Could you check a few things on this model? Use its own coordinates, in mm. A direction names the side the tool comes from. Coordinates: 2 decimals unless noted, no trailing zeros. Order: outer loops, then holes, each group sorted by start corner. A loop starts at its lowest first (then second) coordinate and runs counter-clockwise, first axis right, second up. Notation, with made-up numbers: (72.25, 31) - (90.25, 31) arc R13 ccw to (90.25, 41) - close; hole circle Ø4 at (17.25, 10.5). An arc over 180 degrees is marked (long way). Answer as a JSON object with one key per item and string values. Group by question number.
(1) Will these pins go through, and if not, where does the flat tip stop? P1, Ø6.5, axis at x = 2, z = 2, coming from the +Y side (3 decimals); P2, Ø15, axis at x = 0, z = 0, coming from the -Y side; P3, Ø1, axis at y = 20, z = -20.5, coming from the -X side; P4, Ø11.5, axis at x = -218, z = -24, coming from the +Y side.
(2) Imagine slicing it at D-D, the plane x = -274.5. Write out the boundary of the cut face in (y, z).
(3) Imagine slicing it at B-B, the plane x = -215. Write out the boundary of the cut face in (y, z), and give its area (3 significant figures).
(4) Which directions (+Z, -Z, +X, -X, +Y, -Y) give clear straight access to the entire face, cutting with the end or side of a thin tool? Please do faces 1 (the flat face through (-152.4, 0, -19)), 2 (the flat face through (-255, 0, -50.8)), 3 (the flat face through (-355.6, 0, -19)).
(5) Imagine slicing it at C-C, the plane x = -107.5. Write out the boundary of the cut face in (y, z), and give its area (3 significant figures).
(6) Please list where these lines run through material, in increasing order: probe 1 along X at (y, z) = (-5.5, -23); probe 2 along X at (y, z) = (-14, -21); probe 3 along Z at (x, y) = (-151, 11.5).
from build123d import *

# Parameters (mm, degrees)
F1_DEPTH      = 31.75
F1_DEPTH_BACK = 31.75
F2_DEPTH      = 25.4
F2_DEPTH_BACK = 25.4
F3_R          = 6.35
F4_DEPTH      = 15.875
F5_R          = 6.35
F6_DEPTH      = 15.875


with BuildPart() as f1:
    # F0 (on Front) → F1 (new body, two sides)
    with BuildSketch(Plane.XZ) as f1_sk:
        with BuildLine():
            Line((0, -11.055585), (0, -6.35))
            ThreePointArc((0, -6.35), (4.490128, 4.490128), (-6.35, 0))
            Line((-6.35, 0), (-23.488146, 0))
            ThreePointArc((-23.488146, 0), (-25.145368, -0.220064), (-26.687727, -0.865004))
            Line((-26.687727, -0.865004), (-76.2, -29.747163))
            Line((-76.2, -29.747163), (-82.599162, -31.75))
            Line((-82.599162, -31.75), (-120.65, -31.75))
            ThreePointArc((-120.65, -31.75), (-123.825, -32.600739), (-126.149261, -34.925))
            ThreePointArc((-126.149261, -34.925), (-128.473523, -37.249261), (-131.648523, -38.1))
            Line((-131.648523, -38.1), (-152.4, -38.1))
            Line((-152.4, -38.1), (-355.6, -38.1))
            Line((-355.6, -38.1), (-374.65, -38.1))
            ThreePointArc((-374.65, -38.1), (-379.140128, -39.959872), (-381, -44.45))
            ThreePointArc((-381, -44.45), (-379.140128, -48.940128), (-374.65, -50.8))
            Line((-374.65, -50.8), (-131.648523, -50.8))
            ThreePointArc((-131.648523, -50.8), (-128.473523, -51.650739), (-126.149261, -53.975))
            ThreePointArc((-126.149261, -53.975), (-123.825, -56.299261), (-120.65, -57.15))
            Line((-120.65, -57.15), (-76.2, -57.15))
            Line((-76.2, -57.15), (-69.800838, -55.419992))
            Line((-69.800838, -55.419992), (-3.150419, -16.540581))
            ThreePointArc((-3.150419, -16.540581), (-0.843647, -14.218271), (0, -11.055585))
        make_face()
        with BuildLine():
            ThreePointArc((-4.7625, 0), (0, 4.7625), (4.7625, 0))
            ThreePointArc((4.7625, 0), (0, -4.7625), (-4.7625, 0))
        make_face(mode=Mode.SUBTRACT)
    extrude(amount=F1_DEPTH)
    extrude(f1_sk.sketch, amount=-F1_DEPTH_BACK)

    # F0 (on Front) → F2 (join, two sides)
    with BuildSketch(Plane.XZ) as f2_sk:
        with BuildLine():
            ThreePointArc((-4.7625, 0), (0, -4.7625), (4.7625, 0))
            ThreePointArc((4.7625, 0), (0, 4.7625), (-4.7625, 0))
        make_face()
        with BuildLine():
            Line((0, -11.055585), (0, -6.35))
            ThreePointArc((0, -6.35), (4.490128, 4.490128), (-6.35, 0))
            Line((-6.35, 0), (-23.488146, 0))
            ThreePointArc((-23.488146, 0), (-25.145368, -0.220064), (-26.687727, -0.865004))
            Line((-26.687727, -0.865004), (-76.2, -29.747163))
            Line((-76.2, -29.747163), (-82.599162, -31.75))
            Line((-82.599162, -31.75), (-120.65, -31.75))
            ThreePointArc((-120.65, -31.75), (-123.825, -32.600739), (-126.149261, -34.925))
            ThreePointArc((-126.149261, -34.925), (-128.473523, -37.249261), (-131.648523, -38.1))
            Line((-131.648523, -38.1), (-152.4, -38.1))
            Line((-152.4, -38.1), (-355.6, -38.1))
            Line((-355.6, -38.1), (-374.65, -38.1))
            ThreePointArc((-374.65, -38.1), (-379.140128, -39.959872), (-381, -44.45))
            ThreePointArc((-381, -44.45), (-379.140128, -48.940128), (-374.65, -50.8))
            Line((-374.65, -50.8), (-131.648523, -50.8))
            ThreePointArc((-131.648523, -50.8), (-128.473523, -51.650739), (-126.149261, -53.975))
            ThreePointArc((-126.149261, -53.975), (-123.825, -56.299261), (-120.65, -57.15))
            Line((-120.65, -57.15), (-76.2, -57.15))
            Line((-76.2, -57.15), (-69.800838, -55.419992))
            Line((-69.800838, -55.419992), (-3.150419, -16.540581))
            ThreePointArc((-3.150419, -16.540581), (-0.843647, -14.218271), (0, -11.055585))
        make_face()
        with BuildLine():
            ThreePointArc((-4.7625, 0), (0, 4.7625), (4.7625, 0))
            ThreePointArc((4.7625, 0), (0, -4.7625), (-4.7625, 0))
        make_face(mode=Mode.SUBTRACT)
        with BuildLine():
            Line((-355.6, -38.1), (-152.4, -38.1))
            Line((-152.4, -38.1), (-152.4, 0))
            Line((-152.4, 0), (-220.398958, 0))
            ThreePointArc((-220.398958, 0), (-226.142749, -1.926679), (-229.562879, -6.927273))
            ThreePointArc((-229.562879, -6.927273), (-254, -25.4), (-278.437121, -6.927273))
            ThreePointArc((-278.437121, -6.927273), (-281.857251, -1.926679), (-287.601042, 0))
            Line((-287.601042, 0), (-355.6, 0))
            Line((-355.6, 0), (-355.6, -38.1))
        make_face()
    extrude(amount=F2_DEPTH)
    extrude(f2_sk.sketch, amount=-F2_DEPTH_BACK)

    # F3 (on face) → F4 (cut)
    with BuildSketch(Plane(origin=(0, 31.75, 0), x_dir=(-1, 0, 0), z_dir=(0, 1, 0))):
        Circle(F3_R)
    extrude(amount=-F4_DEPTH, mode=Mode.SUBTRACT)

    # F5 (on face) → F6 (cut)
    with BuildSketch(Plane.XZ.offset(31.75)):
        Circle(F5_R)
    extrude(amount=-F6_DEPTH, mode=Mode.SUBTRACT)


solid = f1.part
Result set:
{
 "1": {"P1": "stops at y = 15.875", "P2": "stops at y = -31.75", "P3": "stops at x = -355.6", "P4": "stops at y = 25.4"},
 "2": {"outline": "(-31.75, -50.8) - (31.75, -50.8) - (31.75, -38.1) - (25.4, -38.1) - (25.4, -15) - (-25.4, -15) - (-25.4, -38.1) - (-31.75, -38.1) - close"},
 "3": {"outline": "(-31.75, -50.8) - (31.75, -50.8) - (31.75, -38.1) - (25.4, -38.1) - (25.4, 0) - (-25.4, 0) - (-25.4, -38.1) - (-31.75, -38.1) - close", "area": "2,740 mm^2"},
 "4": {"face 1": "+Z, +Y, -Y", "face 2": "-Z, -X, +Y, -Y", "face 3": "+Z, -X, +Y, -Y"},
 "5": {"outline": "(-31.75, -57.15) - (31.75, -57.15) - (31.75, -31.75) - (-31.75, -31.75) - close", "area": "1,610 mm^2"},
 "6": {"probe 1": "x = -355.6 to -264.78, -243.22 to -152.4, -64.63 to -14.22", "probe 2": "x = -355.6 to -268.29, -239.71 to -152.4, -61.2 to -10.8", "probe 3": "z = -50.8 to -38.1"}
}
